```python
from build123d import *

# Parameters (mm, degrees)
SKETCH1_W           = 60
SKETCH1_H           = 65
BOSS_EXTRUDE1_DEPTH = 8
SKETCH2_R           = 19.05
CUT_EXTRUDE1_DEPTH  = 1.6
SKETCH3_R           = 3.5
CUT_EXTRUDE2_DEPTH  = 7.4
SKETCH4_W           = 60
SKETCH4_H           = 8
BOSS_EXTRUDE2_DEPTH = 104.05
FILLET1_R           = 10
SKETCH5_W           = 60
SKETCH5_H           = 8
BOSS_EXTRUDE3_DEPTH = 25
BOSS_EXTRUDE4_DEPTH = 5


with BuildPart() as part:
    # Sketch1 → Boss-Extrude1 (new body)
    with BuildSketch(Plane(origin=(0, 0, 0), x_dir=(1, 0, 0), z_dir=(0, 1, 0))):
        Rectangle(SKETCH1_W, SKETCH1_H)
    extrude(amount=BOSS_EXTRUDE1_DEPTH)

    # Sketch2 → Cut-Extrude1 (cut)
    with BuildSketch(Plane.XZ):
        Circle(SKETCH2_R)
    extrude(amount=-CUT_EXTRUDE1_DEPTH, mode=Mode.SUBTRACT)

    # Sketch3 → Cut-Extrude2 (cut, through all)
    with BuildSketch(Plane.XZ.offset(-1.6)):
        Circle(SKETCH3_R)
    extrude(amount=-CUT_EXTRUDE2_DEPTH, mode=Mode.SUBTRACT)

    # Sketch4 → Boss-Extrude2 (add)
    with BuildSketch(Plane(origin=(0, 8, 0), x_dir=(1, 0, 0), z_dir=(0, 1, 0))):
        with Locations((0, 36.5)):
            Rectangle(SKETCH4_W, SKETCH4_H)
    extrude(amount=-BOSS_EXTRUDE2_DEPTH)

    # Fillet1
    fillet1_edges = [part.edges().sort_by_distance(p)[0] for p in [
        (-30, 4, 32.5),
        (30, 4, 32.5),
    ]]
    fillet(fillet1_edges, radius=FILLET1_R)

    # Sketch5 → Boss-Extrude3 (add)
    with BuildSketch(Plane(origin=(0, 0, -40.5), x_dir=(-1, 0, 0), z_dir=(0, 0, -1))):
        with Locations((0, -92.05)):
            Rectangle(SKETCH5_W, SKETCH5_H)
    extrude(amount=BOSS_EXTRUDE3_DEPTH)

    # Sketch6 → Boss-Extrude4 (add)
    with BuildSketch(Plane(origin=(30, 0, 0), x_dir=(0, 0, -1), z_dir=(1, 0, 0))):
        Polygon((40.5, 8), (65.5, -88.05), (40.5, -88.05), align=None)
    boss_extrude4 = extrude(amount=-BOSS_EXTRUDE4_DEPTH)

    # Mirror1: Boss-Extrude4 across plane
    add(boss_extrude4.mirror(Plane(origin=(0, 0, 0), x_dir=(0, 0, 1), z_dir=(1, 0, 0))))


solid = part.part
```
Verification items for the finished model (mm, model axes). A direction names the side the tool comes from. Round coordinates to 2 decimals unless told otherwise and drop trailing zeros. Order: outer loops, then holes, each group sorted by start corner. A loop starts at its lowest first (then second) coordinate and runs counter-clockwise, first axis right, second up. Notation, with made-up numbers: (88, 52) -> (110, 52) arc R20 ccw to (110, 87) -> close; hole circle Ø5 at (63, 1.25). An arc over 180 degrees is marked (long way). Put each result on its own line as item: value. Start each with the question number.
(1) Section check D-D (z = -14.5). Enter the section's corners in (x, y), then the cut area to 3 significant figures.
(2) Section check B-B (x = 0). Enter the section's corners in (y, z), then the cut area to 3 significant figures.
(3) Tool access check on faces 1 (the face through (-14, 0, -15)), 2 (the face through (-25, -61, -48)), 3 (the face through (4, 1.6, 0)), 4 (the face through (3.233, 4.755, -1.341)). Record the directions out of +Z, -Z, +X, -X, +Y, -Y that give a thin tool (end or side, any length) a straight path to the whole face; none if there is none.
(4) Depth check by flat-ended pin: pin 1 Ø1.5 at (x, y) = (-18, -10.5) entering from -Z; pin 2 Ø19 at (x, z) = (5, -6.5) entering from -Y; pin 3 Ø7.5 at (x, z) = (-9, -58) entering from +Y. Enter the tip coordinate at first touch or a pass-through.
(5) Material ranges on line 1 along Z through (x, y) = (0, 5.25); line 2 along Y through (x, z) = (-19.5, 3); line 3 along Z through (x, y) = (3, -78), recorded low to high.
(6) Section check C-C (y = -30). Enter the section's corners in (x, z), then the cut area to 3 significant figures.
(7) Section check A-A (z = 0). Enter the section's corners in (x, y), then the cut area to 3 significant figures.
(8) Draft check along X on faces 5 (the face through (0, -47, -32.5)), 6 (the face through (25, -61, -48)), 7 (the face through (0, -39, -40.5)), 8 (the face through (30, -44, -38)). Enter one of: +X half, -X half, draft (parallel to the pull), parting line (faces both ways), or undercut.
Completed:
1. outline: (-30, 0) -> (-12.36, 0) -> (-12.36, 1.6) -> (12.36, 1.6) -> (12.36, 0) -> (30, 0) -> (30, 8) -> (-30, 8) -> close
1. area: 440 mm2
2. outline: (-96.05, -65.5) -> (-88.05, -65.5) -> (-88.05, -40.5) -> (8, -40.5) -> (8, -3.5) -> (1.6, -3.5) -> (1.6, -19.05) -> (0, -19.05) -> (0, -32.5) -> (-96.05, -32.5) -> close; (0, 19.05) -> (1.6, 19.05) -> (1.6, 3.5) -> (8, 3.5) -> (8, 32.5) -> (0, 32.5) -> close
2. area: 1,450 mm2
3. face 1: +Z, +X, -X, -Y
3. face 2: -Z, +Y
3. face 3: -Y
3. face 4: +Y, -Y
4. pin 1: stops at z = -40.5
4. pin 2: stops at y = 1.6
4. pin 3: stops at y = -88.05
5. line 1: z = -40.5 to -3.5, 3.5 to 32.5
5. line 2: y = 0 to 8
5. line 3: z = -40.5 to -32.5
6. outline: (-30, -50.39) -> (-25, -50.39) -> (-25, -40.5) -> (25, -40.5) -> (25, -50.39) -> (30, -50.39) -> (30, -32.5) -> (-30, -32.5) -> close
6. area: 579 mm2
7. outline: (-30, 0) -> (-19.05, 0) -> (-19.05, 1.6) -> (-3.5, 1.6) -> (-3.5, 8) -> (-30, 8) -> close; (3.5, 1.6) -> (19.05, 1.6) -> (19.05, 0) -> (30, 0) -> (30, 8) -> (3.5, 8) -> close
7. area: 374 mm2
8. face 5: draft
8. face 6: undercut
8. face 7: undercut
8. face 8: +X half
